from build123d import *
from build123d.topology import SkipClean

# Parameters (mm, degrees)
SKETCH1_R           = 5.75
SKETCH1_R_2         = 1.5
BOSS_EXTRUDE1_DEPTH = 3
BOSS_EXTRUDE2_START = 4
SKETCH2_R           = 3
SKETCH2_R_2         = 1.5
BOSS_EXTRUDE2_DEPTH = 4
BOSS_EXTRUDE3_START = -7
BOSS_EXTRUDE3_DEPTH = 7
SKETCH4_R           = 1.75
SKETCH4_R_2         = 0.8
BOSS_EXTRUDE4_DEPTH = 2.5
BOSS_EXTRUDE5_START = -0.8
SKETCH5_R           = 5.75
BOSS_EXTRUDE5_DEPTH = 0.8


with BuildPart() as part:
    # Sketch1 → Boss-Extrude1 (new body)
    with BuildSketch(Plane(origin=(0, 0, 0), x_dir=(1, 0, 0), z_dir=(0, 1, 0))):
        with Locations(Location((0, 0, 0), (0, 0, 270))):
            Circle(SKETCH1_R)
        with Locations(Location((0, 0, 0), (0, 0, 270))):
            Circle(SKETCH1_R_2, mode=Mode.SUBTRACT)
    extrude(amount=BOSS_EXTRUDE1_DEPTH)

    # Sketch2 → Boss-Extrude2 (add)
    with SkipClean():  # the faces are left unmerged after this step: merging them gives an invalid solid
        with BuildSketch(Plane.XZ.offset(BOSS_EXTRUDE2_START)):
            with Locations(Location((0, 0, 0), (0, 0, 90))):
                Circle(SKETCH2_R)
            with Locations(Location((0, 0, 0), (0, 0, 270))):
                Circle(SKETCH2_R_2, mode=Mode.SUBTRACT)
        extrude(amount=-BOSS_EXTRUDE2_DEPTH)

    # Sketch3 → Boss-Extrude3 (add)
    with BuildSketch(Plane(origin=(0, 3, 0), x_dir=(1, 0, 0), z_dir=(0, 1, 0)).offset(BOSS_EXTRUDE3_START)):
        with BuildLine():
            Line((-0.878196328, -1.216047371), (0.926753921, -1.179460542))
            ThreePointArc((0.926753921, -1.179460542), (0.030399161, -1.499691932), (-0.878196328, -1.216047371))
        make_face()
    extrude(amount=BOSS_EXTRUDE3_DEPTH)

    # Sketch4 → Boss-Extrude4 (add)
    with BuildSketch(Plane(origin=(0, 3, 0), x_dir=(1, 0, 0), z_dir=(0, 1, 0))):
        with Locations(Location((2.83060587, 1.729454153, 0), (0, 0, 270))):
            Circle(SKETCH4_R)
        with Locations(Location((2.83060587, 1.729454153, 0), (0, 0, 270))):
            Circle(SKETCH4_R_2, mode=Mode.SUBTRACT)
    extrude(amount=BOSS_EXTRUDE4_DEPTH)

    # Sketch5 → Boss-Extrude5 (add)
    with BuildSketch(Plane(origin=(0, 3, 0), x_dir=(1, 0, 0), z_dir=(0, 1, 0)).offset(BOSS_EXTRUDE5_START)):
        with Locations(Location((0, 0, 0), (0, 0, 270))):
            Circle(SKETCH5_R)
    extrude(amount=BOSS_EXTRUDE5_DEPTH)


solid = part.part
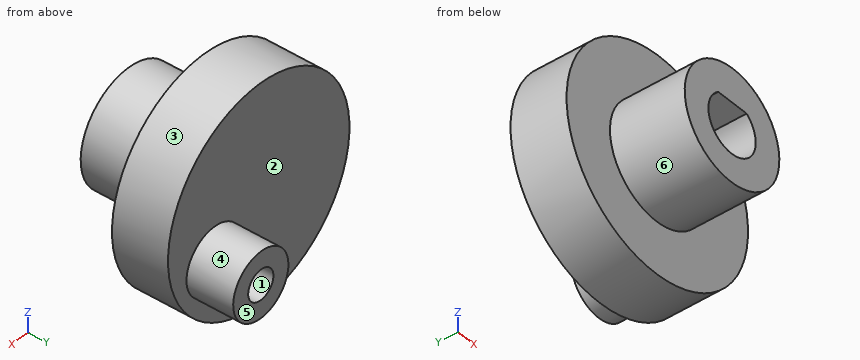
For this review, take the finished solid that the model builds, in its own axes (mm). Face numbers are marked on the shaded views. A direction names the side the tool comes from. Coordinates: 2 decimals unless noted, no trailing zeros. Loops run counter-clockwise (first coordinate to the right, second up) from the corner with the lowest first, then second, coordinate; pieces in that order, holes last. Notation, with made-up numbers: (89, -6.5) - (121, -6.5) arc R30 cw to (121, 19.5) - close; hole circle Ø1 at (-20.5, -37.5). An arc over 180 degrees is marked (long way). Return JSON: item names as keys, results as strings.
Item 1: Take a section at C-C (y = 2.75). Give the boundary of the cut face in (x, z), then the cut area to 3 significant figures.
Determined:
{"outline": "circle Ø11.5 at (0, 0)", "area": "104 mm2"}
Item 2: For the marked faces 4, 5 and 6, list the 3-axis set-ups (+Z, -Z, +X, -X, +Y, -Y) from which the entire face can be reached by the end or side of a thin tool; tool diameter is ignored.
Determined:
{"face 4": "+Y", "face 5": "+Z, -Z, +X, -X, +Y", "face 6": "-Y"}
Item 3: Mouldability with a two-part tool opening along X and no side actions: class the marked faces 1, 2 and 3 as pulls with the +X half, pulls with the -X half, needs draft (parallel to the pull), parting line crosses it, or undercut.
Determined:
{"face 1": "undercut", "face 2": "needs draft", "face 3": "parting line crosses it"}
Item 4: For line 1 (Y direction, x = -3.5, z = 4); line 2 (X direction, y = 1.25, z = -1); line 3 (Z direction, x = -1.25, y = -0.25), list the stretches that pass through material, from the lowest coordinate up.
Determined:
{"line 1": "y = 0 to 3", "line 2": "x = -5.66 to -1.12, 1.12 to 5.66", "line 3": "z = -2.73 to -0.83, 0.83 to 2.73"}
Item 5: Take a section at A-A (y = -3.25). Give the boundary of the cut face in (x, z), then the cut area to 3 significant figures.
Determined:
{"outline": "circle Ø6 at (0, 0); hole (-0.88, 1.22) arc R1.5 ccw (long way) to (0.93, 1.18) - close", "area": "21.6 mm2"}
Item 6: Insertion check: pin 1 (1.8 mm diameter, centred on x = 3, z = -1.5, fed in from +Y); pin 2 (5 mm diameter, centred on x = 4.5, y = -0.5, fed in from -Z); pin 3 (1.5 mm diameter, centred on y = 4, z = -3, fed in from +X); pin 4 (2.5 mm diameter, centred on x = 0, z = 0, fed in from +Y). Each pin has a flat end and moves straight along its axis. Give the tip position at first contact, or say it passes through.
Determined:
{"pin 1": "stops at y = 5.5", "pin 2": "stops at z = -5.37", "pin 3": "stops at x = 4.5", "pin 4": "stops at y = 3"}
Item 7: Take a section at D-D (x = 0). Give the boundary of the cut face in (y, z).
Determined:
{"outline": "(-4, -3) - (0, -3) - (0, -5.75) - (3, -5.75) - (3, 5.75) - (0, 5.75) - (0, 3) - (-4, 3) - (-4, 1.2) - (2.2, 1.2) - (2.2, -1.5) - (-4, -1.5) - close"}
Item 8: Take a section at B-B (z = -3.25). Give the boundary of the cut face in (x, y).
Determined:
{"outline": "(-4.74, 0) - (4.74, 0) - (4.74, 3) - (3.7, 3) - (3.7, 5.5) - (1.96, 5.5) - (1.96, 3) - (-4.74, 3) - close"}
